from build123d import *

# Parameters (mm, degrees)
F0_R     = 9.525
F0_R_2   = 6.35
F1_DEPTH = 66.675
F0_R_3   = 3.175
F2_DEPTH = 84.1502
F3_DEPTH = 17.4752
F4_SIZE  = 1.5875
F5_R     = 3.175
F6_DEPTH = 44.4754


with BuildPart() as f1:
    # F0 (on Top) → F1 (new body)
    with BuildSketch(Plane.XY):
        Circle(F0_R)
        Circle(F0_R_2, mode=Mode.SUBTRACT)
    extrude(amount=F1_DEPTH)

    # F0 (on Top) → F2 (join)
    with BuildSketch(Plane.XY):
        Circle(F0_R_2)
        Circle(F0_R_3, mode=Mode.SUBTRACT)
    extrude(amount=F2_DEPTH)

    # F0 (on Top) → F3 (join)
    with BuildSketch(Plane.XY):
        Circle(F0_R_2)
        Circle(F0_R_3, mode=Mode.SUBTRACT)
    extrude(amount=-F3_DEPTH)

    # F4
    f4_edges = [f1.edges().sort_by_distance(p)[0] for p in [
        (-6.35, 0, -17.4752),
    ]]
    chamfer(f4_edges, length=F4_SIZE)

    # F5 (on face) → F6 (join)
    with BuildSketch(Plane.XY.offset(84.1502)):
        Circle(F5_R)
    extrude(amount=-F6_DEPTH)


solid = f1.part
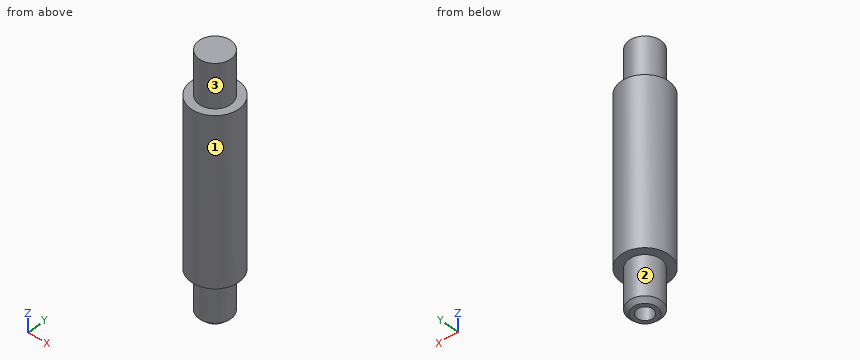
Read the model definition and answer for the solid it produces. Units are mm, in the model's axes. Face numbers are marked on the shaded views. A direction names the side the tool comes from. Coordinates: 2 decimals unless noted, no trailing zeros. Write each loop counter-clockwise with the first axis right and the second up, starting at its lowest first coordinate (ties: lowest second). Pieces come first, ordered by that corner, then holes. Notation, with made-up numbers: (54, -18.5) - (81, -18.5) arc R23 ccw to (81, 2.5) - close; hole circle Ø7 at (11.25, -33.5). An arc over 180 degrees is marked (long way). One line per question, with ' | ' between items.
Q1. Consider L1, parallel to Y at x = 0, z = 1 (3 decimals); L2, parallel to Y at x = 0, z = -3.5 (3 decimals); L3, parallel to Z at x = 7, y = -1.25 (3 decimals). Determine where each line is inside the solid, lowest interval first. Write a range as [from, to].
Result set:
L1: [-9.525, -3.175], [3.175, 9.525] | L2: [-6.35, -3.175], [3.175, 6.35] | L3: [0, 66.675]
Q2. Find section D-D, the plane y = 7.5. Write down the section's boundary in (x, z) (3 decimals), plus the area to 3 significant figures.
Result set:
outline: (-5.872, 0) - (5.872, 0) - (5.872, 66.675) - (-5.872, 66.675) - close | area: 783 mm^2
Q3. Find section C-C, the plane z = 49. Write down the section's boundary in (x, y) (3 decimals).
Result set:
outline: circle Ø19.05 at (0, 0)
Q4. For the marked faces 1, 2 and 3, determine the directions among +Z, -Z, +X, -X, +Y, -Y from which every point of the face is accessible in a straight line to the end or side of a thin tool.
Result set:
face 1: +Z, -Z | face 2: -Z | face 3: +Z
Q5. Each of these flat-tipped pins is pushed along its axis until it touches: P1, Ø1.9, axis at x = 0, y = 1, coming from the -Z side; P2, Ø5, axis at x = -5.5, z = 21, coming from the -Y side; P3, Ø2, axis at x = 6.5, y = -0.5, coming from the -Z side; P4, Ø6, axis at y = 2.5, z = 47.5, coming from the -X side (3 decimals). Where does it stop, or does it pass through?
Result set:
P1: z = 39.67 | P2: y = -9.04 | P3: z = -16.72 | P4: x = -9.525
